For this review, take the finished solid that the model builds, in its own axes (mm). A direction names the side the tool comes from. Round coordinates to 2 decimals unless told otherwise and drop trailing zeros. Order: outer loops, then holes, each group sorted by start corner. A loop starts at its lowest first (then second) coordinate and runs counter-clockwise, first axis right, second up. Notation, with made-up numbers: (33.25, -28) -> (42.25, -28) arc R33 ccw to (42.25, 5) -> close; hole circle Ø8 at (63.25, 26.25). An arc over 180 degrees is marked (long way). Use a Markdown table: item, result. Add a question column.
1) Wall thickness on line 1 along Y through (x, z) = (-0.6, -16); line 2 along X through (y, z) = (-0.25, 14); line 3 along Z through (x, y) = (0.6, 0): over which ranges is each line inside the solid? List them lowest first. Write a range as [from, to].
2) Consider section B-B (z = 16). State the section outline as (x, y) points, plus the area to 3 significant figures.
3) Consider section D-D (z = -16). State the section outline as (x, y) points, plus the area to 3 significant figures.
4) Clearance check with flat-ended pins moving along their axes: P1, Ø2, axis at x = 0.5, y = 1.5, coming from the +Z side; P2, Ø0.9, axis at x = -5, y = -1, coming from the -Z side; P3, Ø3, axis at y = 0.5, z = -6.5, coming from the +X side. State where each tip first meets the part, or that it passes through.
5) Consider section A-A (y = 0). Give the number of separate pieces and of enclosed holes in the cut face, plus the area to 3 significant figures.
6) Draft analysis for pull direction Y (two halves, no side actions). For faces 3 (the face through (3.1, 0, 14)), 4 (the face through (5.33, 0.07, 17.5)), 5 (the face through (5.331, 2.715, 19.699)), state which applies: pulls with the +Y half, pulls with the -Y half, needs draft (parallel to the pull), parting line crosses it, or undercut.
7) Machinability: for faces 1 (the face through (-3.1, 0, 14)), 2 (the face through (7.5, 0, 14)), which of the approach directions +Z, -Z, +X, -X, +Y, -Y give a long, thin tool a straight path to every point of the face, cutting with its end or side? Answer none if there is none.
8) Consider section C-C (x = 5). State the section outline as (y, z) points.
```python
from build123d import *
from build123d.topology import SkipClean

# Parameters (mm, degrees)
SALIENTE_EXTRUIR1_DEPTH    = 2.4
CORTAR_EXTRUIR1_DEPTH      = 21.365657367
CORTAR_EXTRUIR1_DEPTH_BACK = 21.365657367
CROQUIS2_R                 = 1.5
CROQUIS3_R                 = 1.5
SALIENTE_EXTRUIR2_DEPTH    = 7.5
CORTAR_EXTRUIR2_DEPTH      = 3.1
REDONDEO1_R                = 2
REDONDEO2_R                = 1


with BuildPart() as part:
    # Croquis1 → Saliente-Extruir1 (new, symmetric)
    with BuildSketch(Plane(origin=(0, 0, 0), x_dir=(0, 0, -1), z_dir=(1, 0, 0))):
        with BuildLine():
            Line((-19, 3), (19, 3))
            ThreePointArc((19, 3), (19.707106781, 2.707106781), (20, 2))
            Line((20, 2), (20, -2))
            ThreePointArc((20, -2), (19.707106781, -2.707106781), (19, -3))
            Line((19, -3), (-19, -3))
            ThreePointArc((-19, -3), (-19.707106781, -2.707106781), (-20, -2))
            Line((-20, -2), (-20, 2))
            ThreePointArc((-20, 2), (-19.707106781, 2.707106781), (-19, 3))
        make_face()
    extrude(amount=SALIENTE_EXTRUIR1_DEPTH, both=True)

    # Croquis2 → Cortar-Extruir1 (cut, two sides: drawn at the far end of the back side and taken through both)
    with BuildSketch(Plane(origin=(0, 0, 0), x_dir=(0, 0, -1), z_dir=(1, 0, 0)).offset(-CORTAR_EXTRUIR1_DEPTH_BACK)):
        with Locations((-16, 0)):
            Circle(CROQUIS2_R)
        with Locations((16, 0)):
            Circle(CROQUIS2_R)
    extrude(amount=CORTAR_EXTRUIR1_DEPTH + CORTAR_EXTRUIR1_DEPTH_BACK, mode=Mode.SUBTRACT)

    # Croquis3 → Saliente-Extruir2 (add, symmetric)
    with SkipClean():  # the faces are left unmerged after this step: merging them gives an invalid solid
        with BuildSketch(Plane(origin=(0, 0, 0), x_dir=(0, 0, -1), z_dir=(1, 0, 0))):
            with BuildLine():
                Line((-20, 2), (-20, -2))
                ThreePointArc((-20, -2), (-19.707106781, -2.707106781), (-19, -3))
                Line((-19, -3), (-5, -3))
                Line((-5, -3), (-5, 3))
                Line((-5, 3), (-19, 3))
                ThreePointArc((-19, 3), (-19.707106781, 2.707106781), (-20, 2))
            make_face()
            with Locations((-16, 0)):
                Circle(CROQUIS3_R, mode=Mode.SUBTRACT)
        extrude(amount=SALIENTE_EXTRUIR2_DEPTH, both=True)
    add(part.part.scale(1), mode=Mode.REPLACE)  # the faces are merged on a copy

    # Croquis4 → Cortar-Extruir2 (cut, symmetric)
    with BuildSketch(Plane(origin=(0, 0, 0), x_dir=(0, 0, -1), z_dir=(1, 0, 0))):
        with BuildLine():
            Line((-19, 3), (-10, 3))
            Line((-10, 3), (-10, -3))
            Line((-10, -3), (-19, -3))
            ThreePointArc((-19, -3), (-19.707106781, -2.707106781), (-20, -2))
            Line((-20, -2), (-20, 2))
            ThreePointArc((-20, 2), (-19.707106781, 2.707106781), (-19, 3))
        make_face()
    extrude(amount=CORTAR_EXTRUIR2_DEPTH, both=True, mode=Mode.SUBTRACT)

    # Redondeo1
    redondeo1_edges = [part.edges().sort_by_distance(p)[0] for p in [
        (-2.4, 0, 5),
        (2.4, 0, 5),
        (-7.5, 0, 5),
        (7.5, 0, 5),
    ]]
    fillet(redondeo1_edges, radius=REDONDEO1_R)

    # Redondeo2
    redondeo2_edges = [part.edges().sort_by_distance(p)[0] for p in [
        (3.1, 0, 10),
        (-3.1, 0, 10),
    ]]
    fillet(redondeo2_edges, radius=REDONDEO2_R)


solid = part.part
```
Results list:
| question | item | result |
|---|---|---|
| 1 | line 1 | [-3, -1.5], [1.5, 3] |
| 1 | line 2 | [-7.5, -3.1], [3.1, 7.5] |
| 1 | line 3 | [-20, -17.5], [-14.5, 10] |
| 2 | outline | (-7.5, -3) -> (-3.1, -3) -> (-3.1, -1.5) -> (-7.5, -1.5) -> close; (-7.5, 1.5) -> (-3.1, 1.5) -> (-3.1, 3) -> (-7.5, 3) -> close; (3.1, -3) -> (7.5, -3) -> (7.5, -1.5) -> (3.1, -1.5) -> close; (3.1, 1.5) -> (7.5, 1.5) -> (7.5, 3) -> (3.1, 3) -> close |
| 2 | area | 26.4 mm2 |
| 3 | outline | (-2.4, -3) -> (2.4, -3) -> (2.4, -1.5) -> (-2.4, -1.5) -> close; (-2.4, 1.5) -> (2.4, 1.5) -> (2.4, 3) -> (-2.4, 3) -> close |
| 3 | area | 14.4 mm2 |
| 4 | P1 | z = 10 |
| 4 | P2 | z = 5 |
| 4 | P3 | x = 2.4 |
| 5 | separate pieces | 4 |
| 5 | enclosed holes | 0 |
| 5 | area | 243 mm2 |
| 6 | face 3 | needs draft |
| 6 | face 4 | undercut |
| 6 | face 5 | pulls with the +Y half |
| 7 | face 1 | +Z, +Y, -Y |
| 7 | face 2 | +Z, -Z, +X, +Y, -Y |
| 8 | outline | (-3, 5) -> (3, 5) -> (3, 19) arc R1 ccw to (2, 20) -> (-2, 20) arc R1 ccw to (-3, 19) -> close; hole circle Ø3 at (0, 16) |
